from build123d import *

# Parameters (mm, degrees)
BOSS_EXTRUDE1_DEPTH = 10
BOSS_EXTRUDE2_DEPTH = 12
CHAMFER2_SIZE       = 5.5
CHAMFER2_SIZE2      = 9
SKETCH6_W           = 14
SKETCH6_H           = 15
SKETCH6_W_2         = 17
SKETCH6_H_2         = 2.5
SKETCH6_W_3         = 1.5
LPATTERN3_COUNT     = 3
LPATTERN3_PITCH     = 45
SKETCH7_R           = 1.7
CUT_EXTRUDE1_DEPTH  = 10
LPATTERN4_COUNT     = 3
LPATTERN4_PITCH     = 45
LPATTERN5_COUNT     = 2
LPATTERN5_PITCH     = 45
SKETCH8_W           = 10
SKETCH8_H           = 15
SKETCH8_R           = 1.6
BOSS_EXTRUDE3_DEPTH = 5


with BuildPart() as part:
    # Sketch1 → Boss-Extrude1 (new body)
    with BuildSketch(Plane(origin=(0, 0, 0), x_dir=(1, 0, 0), z_dir=(0, 1, 0))):
        with BuildLine():
            Line((0, -11.4), (0, -26))
            Line((0, -26), (22, -26))
            Line((22, -26), (22, 116))
            Line((22, 116), (0, 116))
            Line((0, 116), (0, 101.4))
            ThreePointArc((0, 101.4), (11.4, 90), (0, 78.6))
            Line((0, 78.6), (0, 56.4))
            ThreePointArc((0, 56.4), (11.4, 45), (0, 33.6))
            Line((0, 33.6), (0, 11.4))
            ThreePointArc((0, 11.4), (11.4, 0), (0, -11.4))
        make_face()
    extrude(amount=-BOSS_EXTRUDE1_DEPTH)

    # Sketch3 → Boss-Extrude2 (add)
    with BuildSketch(Plane.XZ.offset(10)):
        with BuildLine():
            Line((0, -116), (0, -101.4))
            ThreePointArc((0, -101.4), (11.4, -90), (0, -78.6))
            Line((0, -78.6), (0, -56.4))
            ThreePointArc((0, -56.4), (11.4, -45), (0, -33.6))
            Line((0, -33.6), (0, -11.4))
            ThreePointArc((0, -11.4), (11.4, 0), (0, 11.4))
            Line((0, 11.4), (0, 26))
            Line((0, 26), (5, 26))
            Line((5, 26), (5, 15.619218931))
            ThreePointArc((5, 15.619218931), (16.4, 0), (5, -15.619218931))
            Line((5, -15.619218931), (5, -29.380781069))
            ThreePointArc((5, -29.380781069), (16.4, -45), (5, -60.619218931))
            Line((5, -60.619218931), (5, -74.380781069))
            ThreePointArc((5, -74.380781069), (16.4, -90), (5, -105.619218931))
            Line((5, -105.619218931), (5, -116))
            Line((5, -116), (0, -116))
        make_face()
    extrude(amount=BOSS_EXTRUDE2_DEPTH)

    # Chamfer2
    chamfer2_edges = [part.edges().sort_by_distance(p)[0] for p in [
        (22, -10, -45),
    ]]
    chamfer2_side = [part.faces().sort_by_distance(p)[0] for p in [
        (6.430139853, -10, 20.809609465),
    ]]
    chamfer(chamfer2_edges, length=CHAMFER2_SIZE, length2=CHAMFER2_SIZE2, reference=chamfer2_side[0])

    # Sketch6 → Cut-Revolve6 (revolve, cut)
    with BuildSketch(Plane.ZY):
        with Locations((-83, -18.5)):
            Rectangle(SKETCH6_W, SKETCH6_H)
        Polygon((-90, -11), (-76, -11), (-73, -8), (-73, -2.5), (-90, -2.5), align=None)
        with Locations((-81.5, -1.25)):
            Rectangle(SKETCH6_W_2, SKETCH6_H_2)
        with Locations((-72.25, -1.25)):
            Rectangle(SKETCH6_W_3, SKETCH6_H_2)
    cut_revolve6 = revolve(axis=Axis((0, 0, -90), (0, -1, 0)), mode=Mode.SUBTRACT)

    # LPattern3: Cut-Revolve6 ×3
    with Locations(*[(0, 0, i * LPATTERN3_PITCH) for i in range(1, LPATTERN3_COUNT)]):
        add(cut_revolve6, mode=Mode.SUBTRACT)

    # Sketch7 → Cut-Extrude1 (cut)
    with BuildSketch(Plane(origin=(5, 0, 0), x_dir=(0, 0, -1), z_dir=(1, 0, 0))):
        with Locations((67.5, -13)):
            Circle(SKETCH7_R)
    cut_extrude1 = extrude(amount=-CUT_EXTRUDE1_DEPTH, mode=Mode.SUBTRACT)

    # LPattern4: Cut-Extrude1 ×3
    with Locations(*[(0, 0, i * LPATTERN4_PITCH) for i in range(1, LPATTERN4_COUNT)]):
        add(cut_extrude1, mode=Mode.SUBTRACT)

    # LPattern5: Cut-Extrude1 ×2
    with Locations(*[(0, 0, -i * LPATTERN5_PITCH) for i in range(1, LPATTERN5_COUNT)]):
        add(cut_extrude1, mode=Mode.SUBTRACT)

    # Sketch8 → Boss-Extrude3 (add)
    with BuildSketch(Plane.XY.offset(26)):
        with Locations((21.5, -7.5)):
            Rectangle(SKETCH8_W, SKETCH8_H)
        with Locations((22.5, -11)):
            Circle(SKETCH8_R, mode=Mode.SUBTRACT)
    extrude(amount=-BOSS_EXTRUDE3_DEPTH)


solid = part.part
Check sheet for the modelled part. Datum: model origin and axes. Units: mm. A direction names the side the tool comes from. Give positions to 0.01 mm unless a question says otherwise; leave off trailing zeros. Order: outer loops, then holes, each group sorted by start corner. A loop starts at its lowest first (then second) coordinate and runs counter-clockwise, first axis right, second up. Notation, with made-up numbers: M 64.5,-14.75 L 100.5,-14.75 A8 ccw 100.5,-7.75 Z; hole C 29,9.25 d8. An arc over 180 degrees is marked long. Answer as CSV lines item,"result". Start each with the question number.
Item 1: Gauge pin test, flat ends, axial feed: P1, Ø0.5, axis at y = -0.5, z = -51.5, coming from the +X side; P2, Ø5, axis at y = -17.5, z = -110.5, coming from the +X side; P3, Ø9.5, axis at x = 7, z = 8, coming from the +Y side; P4, Ø9.5, axis at x = 8.5, z = -46.5, coming from the +Y side (1 decimal). Record the tip position at first contact, or that the pin passes through.
Item 2: Cross-section at C-C on y = -18. Enter the section's corners in (x, z), plus the area to 3 significant figures.
Item 3: Mould release check, pull along Z, two halves, no side actions. Record for faces 1 (the face through (9, -6, -116)), 2 (the face through (14.184, -10.812, -90.312)), 3 (the face through (16.5, -13, 24)), 4 (the face through (14.184, -10.812, -45.312)): +Z half, -Z half, draft (parallel to the pull), parting line (faces both ways), or undercut.
Item 4: Thickness scan on line 1 (Z direction, x = 10.75, y = -1.5); line 2 (Y direction, x = 1.1, z = -67.5); line 3 (Z direction, x = 9.5, y = -6). Record the ranges inside material, lowest first. Write a range as [from, to].
Item 5: Tool access check on faces 5 (the face through (5, -16, 21)), 6 (the face through (5, -16, -111)), 7 (the face through (2.535, -11.567, 21.586)), 8 (the face through (18.496, -1.232, -45.407)), 9 (the face through (5, -16, -22)). Record the directions out of +Z, -Z, +X, -X, +Y, -Y that give a thin tool (end or side, any length) a straight path to the whole face; none if there is none.
Item 6: Cross-section at D-D on x = 10.75. State how many separate pieces and enclosed holes the cut face has, plus the area to 3 significant figures.
Item 7: Cross-section at A-A on z = -67.5. Enter the section's corners in (x, y).
Item 8: Cross-section at B-B on z = -45. Enter the section's corners in (x, y), plus the area to 3 significant figures.
Established:
1,P1,"stops at x = 22"
1,P2,"stops at x = 5"
1,P3,"stops at y = -9.62"
1,P4,"passes through"
2,outline,"M 0,-116 L 5,-116 L 5,-105.62 A16.4 ccw 5,-74.38 L 5,-60.62 A16.4 ccw 5,-29.38 L 5,-15.62 A16.4 ccw 5,15.62 L 5,26 L 0,26 L 0,14 A14 cw 0,-14 L 0,-31 A14 cw 0,-59 L 0,-76 A14 cw 0,-104 Z"
2,area,"570 mm^2"
3,face 1,"-Z half"
3,face 2,"undercut"
3,face 3,"draft"
3,face 4,"undercut"
4,line 1,"z = [-116, -105.06], [-74.94, -60.06], [-29.94, -15.06], [15.06, 26]"
4,line 2,"y = [-22, -14.7], [-11.3, 0]"
4,line 3,"z = [-116, -104.1], [-75.9, -59.1], [-30.9, -14.1], [14.1, 26]"
5,face 5,"+Z, -Y"
5,face 6,"-Z, +X, -Y"
5,face 7,"-X"
5,face 8,"-X, +Y"
5,face 9,"+X, -Y"
6,separate pieces,"4"
6,enclosed holes,"0"
6,area,"859 mm^2"
7,outline,"M 0,-22 L 5,-22 L 5,-14.7 L 0,-14.7 Z; M 0,-11.3 L 5,-11.3 L 5,-10 L 16.5,-10 L 22,-1 L 22,0 L 0,0 Z"
8,outline,"M 14,-22 L 16.4,-22 L 16.4,-10 L 16.5,-10 L 22,-1 L 22,0 L 18.5,0 L 18.5,-2.5 L 17,-2.5 L 17,-8 L 14,-11 Z"
8,area,"51.8 mm^2"
